from build123d import *

# Parameters (mm, degrees)
EXTRUDE_1_DEPTH          = 5
CUT_EXTRUDE_1_DEPTH      = 1202.322110811
CUT_EXTRUDE_1_DEPTH_BACK = 1202.322110811
EXTRUDE_2_DEPTH          = 10


with BuildPart() as part:
    # Эскиз11 → Бобышка-Вытянуть1 (new, symmetric)
    with BuildSketch(Plane.XY):
        with BuildLine():
            Line((636.463912705, 976.146466683), (700.205604925, 770.085305884))
            add(Edge.make_bspline(
                [(700.205604925, 770.085305884), (141.848194954, 128.23481722), (116.561380271, 120.122243094), (-589.536273057, 282.297875154)],
                knots=[0, 0, 0, 0, 1, 1, 1, 1], degree=3))
            Line((-589.536273057, 282.297875154), (-589.536273057, 976.146466683))
            Line((-589.536273057, 976.146466683), (636.463912705, 976.146466683))
        make_face()
    extrude(amount=EXTRUDE_1_DEPTH, both=True)

    # Эскиз12 → Вырез-Вытянуть1 (cut, two sides: drawn at the far end of the back side and taken through both)
    with BuildSketch(Plane.XY.offset(-CUT_EXTRUDE_1_DEPTH_BACK)):
        Polygon((-700.700191259, 528.942112061), (706.16734826, 911.673616779), (340.903623972, 1222.525422138), (-820.682545159, 1079.972181823), align=None)
    extrude(amount=CUT_EXTRUDE_1_DEPTH + CUT_EXTRUDE_1_DEPTH_BACK, mode=Mode.SUBTRACT)


with BuildPart() as cut_extrude_1_piece_1:
    # of the separate pieces the step leaves, piece 1, a body of its own (cut_extrude_1_pieces)
    add(part.part.solids().sort_by_distance((660.269941789, 899.187449498, 5))[0])

    # Эскиз14 → Бобышка-Вытянуть2 (add)
    with BuildSketch(Plane(origin=(0, 0, -5), x_dir=(-1, 0, 0), z_dir=(0, 0, -1))):
        with BuildLine():
            Line((1133.941311309, 411.08096229), (589.536273057, 282.297875154))
            add(Edge.make_bspline(
                [(-637.785646163, 672.312444588), (-248.934023891, 179.435642483), (-152.966629698, 110.557627429), (589.536273057, 282.297875154)],
                knots=[0, 0, 0, 0, 1, 1, 1, 1], degree=3))
            Line((-637.785646163, 672.312444588), (-844.917078579, 949.419809347))
            Line((-844.917078579, 949.419809347), (-660.269941789, 899.187449498))
            Line((-660.269941789, 899.187449498), (1133.941311309, 411.08096229))
        make_face()
    extrude(amount=-EXTRUDE_2_DEPTH)


with BuildPart() as cut_extrude_1_piece_2:
    # of the separate pieces the step leaves, piece 2, a body of its own (cut_extrude_1_pieces)
    add(part.part.solids().sort_by_distance((636.463912705, 976.146466683, -5))[0])


solid = cut_extrude_1_piece_1.part
Geometry: final body of the model. Coordinates: model frame, mm. Round coordinates to 2 decimals unless told otherwise and drop trailing zeros. Order: outer loops, then holes, each group sorted by start corner. A loop starts at its lowest first (then second) coordinate and runs counter-clockwise, first axis right, second up. Notation, with made-up numbers: (58, 79.5) - (102, 79.5) arc R14 ccw to (102, 87.5) - close; hole circle Ø3 at (-36.5, 4). An arc over 180 degrees is marked (long way). Write each question's results on one line, items separated by ' | '.
Item 1: First-contact query: pin 1 Ø6 at (x, z) = (-271.5, -0.5) entering from +Y; pin 2 Ø4 at (y, z) = (525, -2) entering from +X. Flat tips, straight axial feed; report the tip coordinate or a pass-through.
Completed:
pin 1: y = 646.52 | pin 2: x = 520.67
Item 2: Section B-B, the plane y = 794. Return the cut outline in (x, z), and give its area (3 significant figures).
Completed:
outline: (273.62, -5) - (728.74, -5) - (728.74, 5) - (273.62, 5) - close | area: 4,550 mm^2
Item 3: Material intervals for line 1 along Y through (x, z) = (-458.5, 0); line 2 along Y through (x, z) = (71.5, -4.25), sorted ascending. Write a range as [from, to].
Completed:
line 1: [252.6, 594.83] | line 2: [206.49, 739.02]
Item 4: Section A-A, the plane y = 872.5. Return the cut outline in (x, z), and give its area (3 significant figures).
Completed:
outline: (562.17, -5) - (787.42, -5) - (787.42, 5) - (562.17, 5) - close | area: 2,250 mm^2
